Can you work these out from the drawing? Everything is in mm from the part's minimum corner. A direction names the side the tool comes from. Coordinates: 2 decimals unless noted, no trailing zeros. Loops run counter-clockwise (first coordinate to the right, second up) from the corner with the lowest first, then second, coordinate; pieces in that order, holes last.
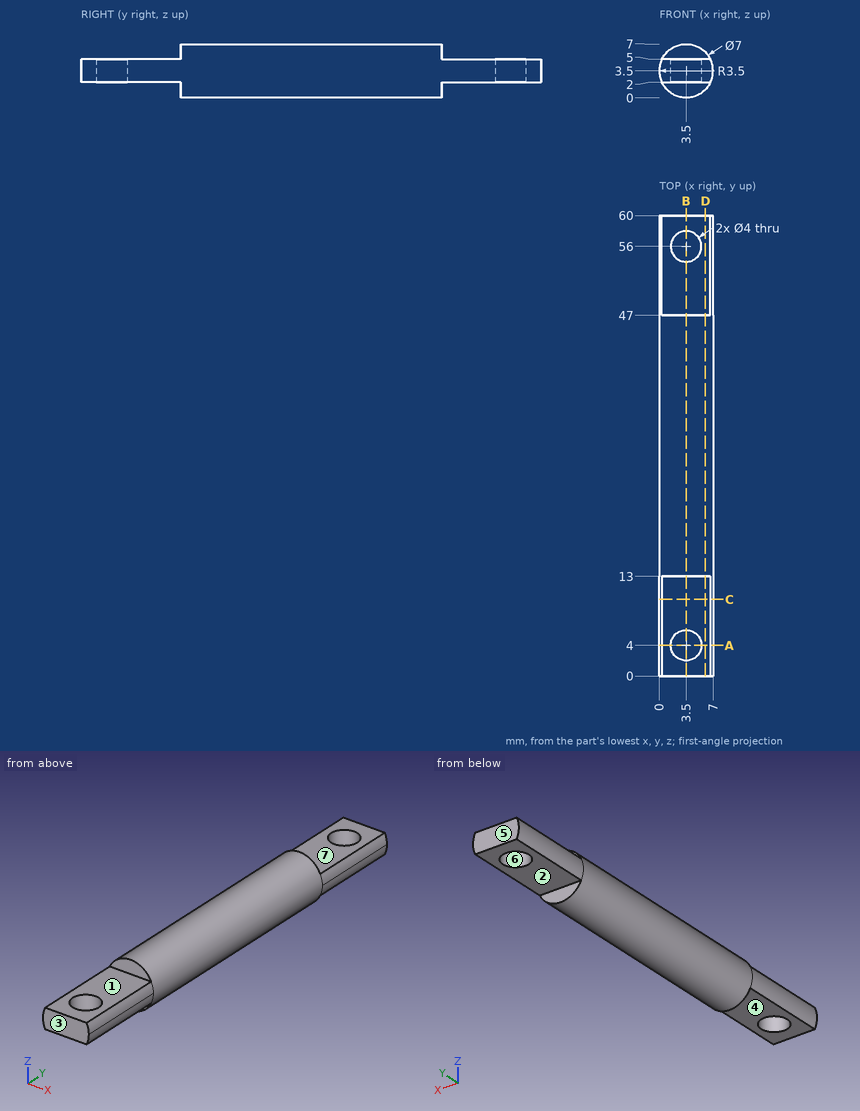
(1) Imagine slicing it at C-C, the plane y = 10. Write out the boundary of the cut face in (x, z), and give its area (3 significant figures).
Answers:
outline: (0.34, 2) - (6.66, 2) arc R3.5 ccw to (6.66, 5) - (0.34, 5) arc R3.5 ccw to start
area: 20.3 mm2
(2) Which directions (+Z, -Z, +X, -X, +Y, -Y) give clear straight access to the entire face, cutting with the end or side of a thin tool? Please do the marked faces 1, 2, 3 and 4.
Answers:
face 1: +Z, +X, -X, -Y
face 2: -Z, +X, -X, +Y
face 3: +Z, -Z, +X, -X, -Y
face 4: -Z, +X, -X, -Y
(3) We'd pull the mould along Y, two halves only. Please class the marked faces 5, 6 and 7: +Y half, -Y half, draft (parallel to the pull), parting line (faces both ways), or undercut.
Answers:
face 5: +Y half
face 6: undercut
face 7: draft
(4) Imagine slicing it at B-B, the plane x = 3.5. Write out the boundary of the cut face in (y, z).
Answers:
outline: (0, 2) - (2, 2) - (2, 5) - (0, 5) - close; (6, 2) - (13, 2) - (13, 0) - (47, 0) - (47, 2) - (54, 2) - (54, 5) - (47, 5) - (47, 7) - (13, 7) - (13, 5) - (6, 5) - close; (58, 2) - (60, 2) - (60, 5) - (58, 5) - close
(5) Imagine slicing it at A-A, the plane y = 4. Write out the boundary of the cut face in (x, z), and give its area (3 significant figures).
Answers:
outline: (0.34, 2) - (1.5, 2) - (1.5, 5) - (0.34, 5) arc R3.5 ccw to start; (5.5, 2) - (6.66, 2) arc R3.5 ccw to (6.66, 5) - (5.5, 5) - close
area: 8.34 mm2
(6) Imagine slicing it at D-D, the plane x = 6. Write out the boundary of the cut face in (y, z), and give its area (3 significant figures).
Answers:
outline: (0, 2) - (13, 2) - (13, 1.05) - (47, 1.05) - (47, 2) - (60, 2) - (60, 5) - (47, 5) - (47, 5.95) - (13, 5.95) - (13, 5) - (0, 5) - close
area: 245 mm2
(7) I need wall thicknesses on probe 1 along Y at (x, z) = (3.5, 3.9); probe 2 along Y at (x, z) = (1.75, 4.5); probe 3 along Y at (x, z) = (2.25, 1.5). Which ranges of each line are inside material? Lowest first, please.
Answers:
probe 1: y = 0 to 2, 6 to 54, 58 to 60
probe 2: y = 0 to 3.03, 4.97 to 55.03, 56.97 to 60
probe 3: y = 13 to 47
(8) For pin 1 (0.6 mm diameter, centred on x = 3.5, z = 0.5, fed in from +Y); pin 2 (3 mm diameter, centred on y = 15, z = 1, fed in from +X); pin 3 (3 mm diameter, centred on x = 3, y = 7, fed in from -Z), each with a flat end and sliding along its axis, tell me the tip position at first contact or that it passes through.
Answers:
pin 1: stops at y = 47
pin 2: stops at x = 6.85
pin 3: stops at z = 2
